Build history of the part. All positions in model axes, mm. Coordinates: 2 decimals unless noted, no trailing zeros. Order: outer loops, then holes, each group sorted by start corner. A loop starts at its lowest first (then second) coordinate and runs counter-clockwise, first axis right, second up. Notation, with made-up numbers: (-25.75, 9.5) - (10.25, 9.5) arc R28 cw to (10.25, 41.5) - close; hole circle Ø5 at (80, -30.5). An arc over 180 degrees is marked (long way). Write each question's results on one line, items separated by ' | '. Start each with the question number.
from build123d import *

# Parameters (mm, degrees)
SKETCH1_W                    = 244.475
SKETCH1_H                    = 244.475
MAIN_BODY_DEPTH              = 1.5875
SKETCH2_R                    = 3.175
SKETCH2_R_2                  = 2.286
SCREW_AND_STRING_HOLES_DEPTH = 2.5875
SKETCH4_W                    = 12.7
SKETCH4_H                    = 12.7
LED_HOLES_DEPTH              = 2.5875
EXTERNAL_CABLE_SLOTS_DEPTH   = 2.5875


with BuildPart() as part:
    # Sketch1 → Main Body (new body)
    with BuildSketch(Plane(origin=(0, 0, 0), x_dir=(1, 0, 0), z_dir=(0, 1, 0))):
        with Locations((122.2375, 122.2375)):
            Rectangle(SKETCH1_W, SKETCH1_H)
    extrude(amount=MAIN_BODY_DEPTH)

    # Sketch2 → Screw and String Holes (cut, through all)
    with BuildSketch(Plane(origin=(0, 1.5875, 0), x_dir=(1, 0, 0), z_dir=(0, 1, 0))):
        with Locations((211.1375, 33.3375)):
            Circle(SKETCH2_R)
        with Locations((33.3375, 33.3375)):
            Circle(SKETCH2_R)
        with Locations((33.3375, 211.1375)):
            Circle(SKETCH2_R)
        with Locations((211.1375, 211.1375)):
            Circle(SKETCH2_R)
        with Locations((228.6, 15.875)):
            Circle(SKETCH2_R_2)
        with Locations((15.875, 15.875)):
            Circle(SKETCH2_R_2)
        with Locations((15.875000001, 228.6)):
            Circle(SKETCH2_R_2)
        with Locations((228.6, 228.6)):
            Circle(SKETCH2_R_2)
    extrude(amount=-SCREW_AND_STRING_HOLES_DEPTH, mode=Mode.SUBTRACT)

    # Sketch4 → LED Holes (cut, through all)
    with BuildSketch(Plane(origin=(0, 1.5875, 0), x_dir=(1, 0, 0), z_dir=(0, 1, 0))):
        with Locations((122.2375, 25.4)):
            Rectangle(SKETCH4_W, SKETCH4_H)
        with Locations((25.4, 122.2375)):
            Rectangle(SKETCH4_W, SKETCH4_H)
        with Locations((122.2375, 219.075)):
            Rectangle(SKETCH4_W, SKETCH4_H)
        with Locations((219.075, 122.2375)):
            Rectangle(SKETCH4_W, SKETCH4_H)
    extrude(amount=-LED_HOLES_DEPTH, mode=Mode.SUBTRACT)

    # Sketch5 → External Cable Slots (cut, through all)
    with BuildSketch(Plane(origin=(0, 1.5875, 0), x_dir=(1, 0, 0), z_dir=(0, 1, 0))):
        with BuildLine():
            Line((109.5375, 101.9175), (134.9375, 101.9175))
            ThreePointArc((134.9375, 101.9175), (140.0175, 96.8375), (134.9375, 91.7575))
            Line((134.9375, 91.7575), (109.5375, 91.7575))
            ThreePointArc((109.5375, 91.7575), (104.4575, 96.8375), (109.5375, 101.9175))
        make_face()
        with BuildLine():
            Line((109.5375, 152.7175), (134.9375, 152.7175))
            ThreePointArc((134.9375, 152.7175), (140.0175, 147.6375), (134.9375, 142.5575))
            Line((134.9375, 142.5575), (109.5375, 142.5575))
            ThreePointArc((109.5375, 142.5575), (104.4575, 147.6375), (109.5375, 152.7175))
        make_face()
    extrude(amount=-EXTERNAL_CABLE_SLOTS_DEPTH, mode=Mode.SUBTRACT)


solid = part.part
Item 1: Pull direction Z, two halves, no side cores. Call faces 1 (the flat face through (121, 0, -124)), 2 (the cylindrical face through (35.044, 0.805, -36.015)): released by +Z, released by -Z, zero draft, split by the parting line, or undercut.
Item 2: Slice it at B-B (y = 1.15). Count the separate pieces of the cut face and the enclosed holes in it, then the cut area to 3 significant figures.
Item 3: Slice it at A-A (z = -220.5). Write the cut outline in (x, y) (1 decimal), then the cut area to 3 significant figures.
Item 4: Probe probe 1 along X at (y, z) = (0.25, -122) (3 decimals); probe 2 along Z at (x, y) = (132, 0.75) (1 decimal); probe 3 along Z at (x, y) = (211, 1.2) (3 decimals). List the from-to ranges inside material, lowest first.
Item 5: Flat gauge pins, fed straight in: P1, Ø4, axis at x = 15.875, z = -228.6, coming from the -Y side; P2, Ø7.5, axis at x = 228.6, z = -15.875, coming from the -Y side. Where does each tip first touch, or does it go through?
Resolved:
1) face 1: zero draft | face 2: undercut
2) separate pieces: 1 | enclosed holes: 14 | area: 58,300 mm^2
3) outline: (0, 0) - (115.9, 0) - (115.9, 1.6) - (0, 1.6) - close; (128.6, 0) - (244.5, 0) - (244.5, 1.6) - (128.6, 1.6) - close | area: 368 mm^2
4) probe 1: 0 to 19.05, 31.75 to 212.725, 225.425 to 244.475 | probe 2: -244.5 to -152.7, -142.6 to -101.9, -91.8 to 0 | probe 3: -244.475 to -214.31, -207.965 to -36.51, -30.165 to 0
5) P1: through | P2: y = 0
